The listing builds one solid part. Answer for the finished solid, in the listing's coordinates (mm). Face numbers are marked on the shaded views. A direction names the side the tool comes from. Round coordinates to 2 decimals unless told otherwise and drop trailing zeros. Loops run counter-clockwise (first coordinate to the right, second up) from the corner with the lowest first, then second, coordinate; pieces in that order, holes last. Notation, with made-up numbers: (63, 36) - (113, 36) arc R24 cw to (113, 60) - close; hole circle Ø6 at (62, -39). An arc over 180 degrees is marked (long way). Write item = value, one per line. Start each with the question number.
1) Section D-D, the plane z = 11.5 is taken. Determine the outline of the cut face in (x, y).
2) Section A-A, the plane y = -7.84 is taken. Determine the outline of the cut face in (x, z), and give its area (3 significant figures).
3) Section C-C, the plane z = 2 is taken. Determine the outline of the cut face in (x, y), and give its area (3 significant figures).
4) Given pin 1 Ø11.5 at (y, z) = (-7.84, 0) entering from +X; pin 2 Ø8.5 at (x, z) = (5.5, -4) entering from +Y; pin 3 Ø2 at (y, z) = (4.5, 1) entering from +X; pin 4 Ø14.5 at (y, z) = (4.5, -1) entering from +X, each flat-ended and moving along its own axis, determine where each tip first touches the part or whether it passes through.
5) For a pull along Z with two mould halves and no side action, classify the marked faces 3, 4, 5 and 6 as released by +Z, released by -Z, zero draft, split by the parting line, or undercut.
6) Straight lines are drawn through the part: line 1 along Y through (x, z) = (-7, 0); line 2 along X through (y, z) = (11.75, -6); line 3 along Z through (x, y) = (14, -7.84). For each, find the intervals that lie inside material, in ascending order.
7) Section B-B, the plane x = 11 is taken. Determine the outline of the cut face in (y, z), and give its area (3 significant figures).
8) A tool of negligible diameter and unlimited length cuts with its end or side. For the marked faces 1 and 2, from which of +Z, -Z, +X, -X, +Y, -Y can it reach the whole face along a straight path? Write none if from no direction.
from build123d import *

# Parameters (mm, degrees)
BOSS_EXTRUDE1_DEPTH      = 15
BOSS_EXTRUDE1_DEPTH_BACK = 15
CUT_EXTRUDE1_DEPTH       = 55.4
CUT_EXTRUDE1_DEPTH_BACK  = 30
SKETCH2_R                = 4
SKETCH3_R                = 6.5
CUT_EXTRUDE2_DEPTH       = 18.2


with BuildPart() as part:
    # Sketch1 → Boss-Extrude1 (new, two sides: drawn at the far end of the back side and taken through both)
    with BuildSketch(Plane.XY.offset(-BOSS_EXTRUDE1_DEPTH_BACK)):
        with BuildLine():
            Line((-10, -15.714961024), (-10, 14.285038976))
            Line((-10, 14.285038976), (0, 14.285038976))
            Line((0, 14.285038976), (0, 1))
            ThreePointArc((0, 1), (-0.707106781, -0.707106781), (1, 0))
            Line((1, 0), (18, 0))
            Line((18, 0), (18, -11.84))
            Line((18, -11.84), (19.0754, -11.84))
            Line((19.0754, -11.84), (19.0754, -15.714961024))
            Line((19.0754, -15.714961024), (-10, -15.714961024))
        make_face()
    extrude(amount=BOSS_EXTRUDE1_DEPTH + BOSS_EXTRUDE1_DEPTH_BACK)

    # Sketch2 → Cut-Extrude1 (cut, two sides: drawn at the far end of the back side and taken through both)
    with BuildSketch(Plane(origin=(0, 0, 0), x_dir=(0, 0, -1), z_dir=(1, 0, 0)).offset(-CUT_EXTRUDE1_DEPTH_BACK)):
        with Locations(Location((0, -7.84, 0), (0, 0, 270))):
            Circle(SKETCH2_R)
    extrude(amount=CUT_EXTRUDE1_DEPTH + CUT_EXTRUDE1_DEPTH_BACK, mode=Mode.SUBTRACT)

    # Sketch3 → Cut-Extrude2 (cut)
    with BuildSketch(Plane(origin=(0, 0, 0), x_dir=(0, 0, -1), z_dir=(1, 0, 0))):
        with Locations((0, -7.84)):
            Circle(SKETCH3_R)
    extrude(amount=-CUT_EXTRUDE2_DEPTH, mode=Mode.SUBTRACT)


solid = part.part
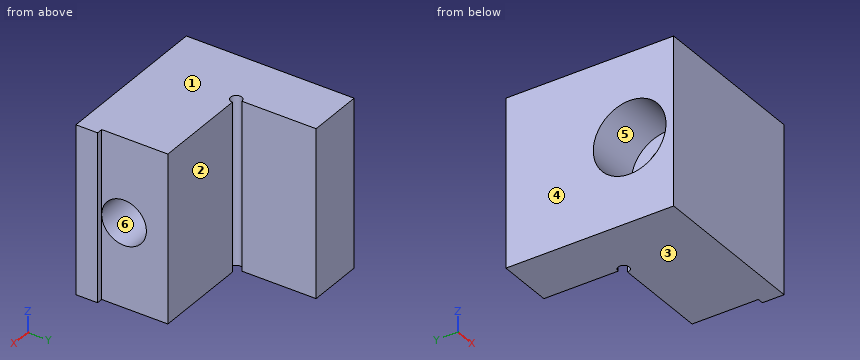
Geometry check:
q1.outline = (-10, -15.71) - (19.08, -15.71) - (19.08, -11.84) - (18, -11.84) - (18, 0) - (1, 0) arc R1 cw (long way) to (0, 1) - (0, 14.29) - (-10, 14.29) - close
q2.outline = (-10, -15) - (18, -15) - (18, -4) - (0, -4) - (0, -6.5) - (-10, -6.5) - close; (-10, 6.5) - (0, 6.5) - (0, 4) - (18, 4) - (18, 15) - (-10, 15) - close
q2.area = 566 mm2
q3.outline = (-10, -15.71) - (19.08, -15.71) - (19.08, -11.84) - (18, -11.84) - (18, -11.3) - (0, -11.3) - (0, -14.02) - (-10, -14.02) - close; (-10, -1.66) - (0, -1.66) - (0, -4.38) - (18, -4.38) - (18, 0) - (1, 0) arc R1 cw (long way) to (0, 1) - (0, 14.29) - (-10, 14.29) - close
q3.area = 336 mm2
q4.pin_1 = 19.08
q4.pin_2 = 0
q4.pin_3 = 0
q4.pin_4 = 18
q5.face_3 = released by -Z
q5.face_4 = zero draft
q5.face_5 = undercut
q5.face_6 = undercut
q6.line_1 = -15.71 to -14.34, -1.34 to 14.29
q6.line_2 = -10 to 0
q6.line_3 = -15 to -4, 4 to 15
q7.outline = (-15.71, -15) - (0, -15) - (0, 15) - (-15.71, 15) - close; hole circle Ø8 at (-7.84, 0)
q7.area = 421 mm2
q8.face_1 = +Z, +X, -X, +Y, -Y
q8.face_2 = +Z, -Z, +X, +Y
